Could you check a few things on this model? Use its own coordinates, in mm. Face numbers are marked on the shaded views. A direction names the side the tool comes from. Coordinates: 2 decimals unless noted, no trailing zeros. Write each loop counter-clockwise with the first axis right and the second up, starting at its lowest first coordinate (ties: lowest second). Pieces come first, ordered by that corner, then holes. Notation, with made-up numbers: M 13.5,37 L 22.5,37 A25 cw 22.5,64 Z; hole C 63.25,66.25 d9. An arc over 180 degrees is marked long. Write item = value, one per line.
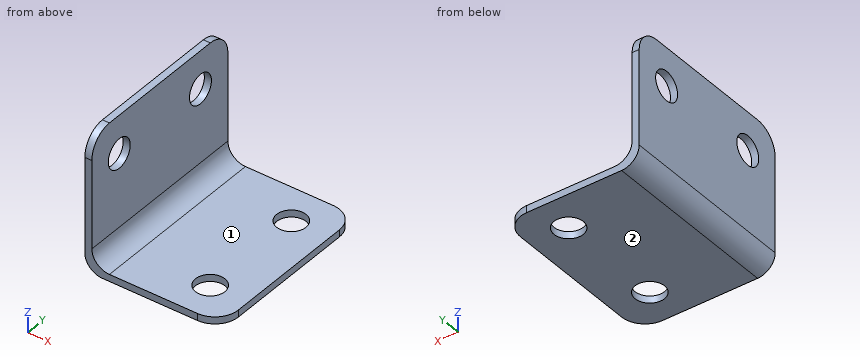
```python
from build123d import *

# Parameters (mm, degrees)
EXTRUDE_1_DEPTH     = 31
SKETCH_2_R          = 2.5
CUT_EXTRUDE_1_DEPTH = 30.5
SKETCH_4_R          = 2.5
CUT_EXTRUDE_2_DEPTH = 30.5


with BuildPart() as part:
    # 草图1 → 凸台-拉伸1 (new body)
    with BuildSketch(Plane(origin=(0, 0, 0), x_dir=(1, 0, 0), z_dir=(0, 1, 0))):
        with BuildLine():
            Line((3, 0), (23.2, 0))
            Line((23.2, 0), (23.2, -1.2))
            Line((23.2, -1.2), (4.2, -1.2))
            ThreePointArc((4.2, -1.2), (2.078679656, -2.078679656), (1.2, -4.2))
            Line((1.2, -4.2), (1.2, -23.2))
            Line((1.2, -23.2), (0, -23.2))
            Line((0, -23.2), (0, -3))
            ThreePointArc((0, -3), (0.878679656, -0.878679656), (3, 0))
        make_face()
    extrude(amount=EXTRUDE_1_DEPTH)

    # 草图2 → 切除-拉伸1 (cut)
    with BuildSketch(Plane.XY.offset(1.2)):
        with BuildLine():
            ThreePointArc((19.2, 31), (22.028427125, 29.828427125), (23.2, 27))
            Line((23.2, 27), (23.2, 31))
            Line((23.2, 31), (19.2, 31))
        make_face()
        with Locations((16.7, 24.75)):
            Circle(SKETCH_2_R)
        with BuildLine():
            Line((23.2, 0), (23.2, 4))
            ThreePointArc((23.2, 4), (22.028427125, 1.171572875), (19.2, 0))
            Line((19.2, 0), (23.2, 0))
        make_face()
        with Locations((16.7, 6.25)):
            Circle(SKETCH_2_R)
    extrude(amount=-CUT_EXTRUDE_1_DEPTH, mode=Mode.SUBTRACT)

    # 草图4 → 切除-拉伸2 (cut)
    with BuildSketch(Plane(origin=(1.2, 0, 1), x_dir=(0, 0, -1), z_dir=(1, 0, 0))):
        with Locations((-15.7, 6.25)):
            Circle(SKETCH_4_R)
        with BuildLine():
            ThreePointArc((-18.2, 0), (-21.028427125, 1.171572875), (-22.2, 4))
            Line((-22.2, 4), (-22.2, 0))
            Line((-22.2, 0), (-18.2, 0))
        make_face()
        with BuildLine():
            Line((-22.2, 31), (-22.2, 27))
            ThreePointArc((-22.2, 27), (-21.028427125, 29.828427125), (-18.2, 31))
            Line((-18.2, 31), (-22.2, 31))
        make_face()
        with Locations((-15.7, 24.75)):
            Circle(SKETCH_4_R)
    extrude(amount=-CUT_EXTRUDE_2_DEPTH, mode=Mode.SUBTRACT)


solid = part.part
```
Item 1: Imagine slicing it at A-A (y = 6.25). Write out the boundary of the cut face in (x, z), and give its area (3 significant figures).
Numbers:
outline = M 0,3 A3 ccw 3,0 L 14.2,0 L 14.2,1.2 L 4.2,1.2 A3 cw 1.2,4.2 L 1.2,14.2 L 0,14.2 Z; M 0,19.2 L 1.2,19.2 L 1.2,23.2 L 0,23.2 Z; M 19.2,0 L 23.2,0 L 23.2,1.2 L 19.2,1.2 Z
area = 42.2 mm²
Item 2: I'm going to push flat-ended pins straight in: P1, Ø5, axis at y = 3.5, z = 19, coming from the -X side; P2, Ø2, axis at y = 9, z = 16, coming from the +X side; P3, Ø4.5, axis at y = 24.75, z = 16.7, coming from the -X side; P4, Ø6, axis at x = 16.7, y = 6.25, coming from the +Z side. Where does each tip first touch, or does it pass through?
Numbers:
P1 = 0
P2 = 1.2
P3 = through
P4 = 1.2
Item 3: Imagine slicing it at C-C (y = 10.5). Write out the boundary of the cut face in (x, z).
Numbers:
outline = M 0,3 A3 ccw 3,0 L 23.2,0 L 23.2,1.2 L 4.2,1.2 A3 cw 1.2,4.2 L 1.2,23.2 L 0,23.2 Z
Item 4: For the marked faces 1 and 2, which set-ups out of +Z, -Z, +X, -X, +Y, -Y let a thin tool reach every point of the face, with its end or its side?
Numbers:
face_1 = +Z, +X, +Y, -Y
face_2 = -Z, +X, -X, +Y, -Y
Item 5: Imagine slicing it at D-D (z = 15.75). Write out the boundary of the cut face in (x, y), and give its area (3 significant figures).
Numbers:
outline = M 0,0 L 1.2,0 L 1.2,3.94 L 0,3.94 Z; M 0,8.56 L 1.2,8.56 L 1.2,22.44 L 0,22.44 Z; M 0,27.06 L 1.2,27.06 L 1.2,31 L 0,31 Z
area = 26.1 mm²
Item 6: Imagine slicing it at B-B (x = 16.7). Write out the boundary of the cut face in (y, z).
Numbers:
outline = M 0,0 L 3.75,0 L 3.75,1.2 L 0,1.2 Z; M 8.75,0 L 22.25,0 L 22.25,1.2 L 8.75,1.2 Z; M 27.25,0 L 31,0 L 31,1.2 L 27.25,1.2 Z
Item 7: If I drill on line 1 along Y through (x, z) = (0.7, 16.7); line 2 along Z through (x, y) = (10, 6.5), over which ranges is the centre line in solid material (lowest first)?
Numbers:
line_1 = 0 to 3.75, 8.75 to 22.25, 27.25 to 31
line_2 = 0 to 1.2
